Model file for the job. Use its own axes, mm. Face numbers are marked on the shaded views. Round coordinates to 2 decimals unless told otherwise and drop trailing zeros. Order: outer loops, then holes, each group sorted by start corner. A loop starts at its lowest first (then second) coordinate and runs counter-clockwise, first axis right, second up. Notation, with made-up numbers: (46, 83.25) - (92, 83.25) arc R14 ccw to (92, 91.25) - close; hole circle Ø10 at (61, 34). An arc over 180 degrees is marked (long way). Answer as CSV lines item,"result". Start each with the question number.
1. Wall check: line 1 along Y through (x, z) = (1.8, 0) (3 decimals); line 2 along Z through (x, y) = (0.8, 0) (3 decimals); line 3 along Y through (x, z) = (0.3, -1.25). Give the ranges that are in metal, low to high. Write a range as [from, to].
2. Pull direction Z, two halves, no side cores. Call the marked faces 1, 2 and 3: released by +Z, released by -Z, zero draft, split by the parting line, or undercut.
3. Band-saw the part on A-A on x = 1.5. List the corners of the cut face in (y, z) (3 decimals), then the cut area to 3 significant figures.
4. Pin check, flat tips, straight feed: pin 1 Ø1.5 at (x, z) = (1.5, -2) entering from -Y; pin 2 Ø1 at (x, y) = (2, -1.5) entering from -Z. Stop position of each tip, or through.
```python
from build123d import *

# Parameters (mm, degrees)
RESSALTO_EXTRUS_O1_DEPTH = 3
FILETE1_R                = 0.2
ESBO_O12_OUTSIDE_W       = 88.106
ESBO_O12_OUTSIDE_H       = 86.648
ESBO_O12_OUTSIDE_R       = 5
CORTE_EXTRUS_O3_DEPTH    = 13
CORTE_EXTRUS_O3_DRAFT    = -70
ESBO_O17_OUTSIDE_W       = 88.106
ESBO_O17_OUTSIDE_H       = 86.648
ESBO_O17_OUTSIDE_R       = 4.994498725
CORTE_EXTRUS_O4_DEPTH    = 13
CORTE_EXTRUS_O4_DRAFT    = -70


with BuildPart() as part:
    # Esboço1 → Ressalto-extrusão1 (new body)
    with BuildSketch(Plane(origin=(0, 0, 0), x_dir=(0, 0, -1), z_dir=(1, 0, 0))):
        Polygon((2.808721651, 5.044245833), (-2.964084209, 4.954547218), (-5.77280586, -0.089698615), (-2.808721651, -5.044245833), (2.964084209, -4.954547218), (5.77280586, 0.089698615), align=None)
    extrude(amount=RESSALTO_EXTRUS_O1_DEPTH)

    # Esboço11 → Furo roscado de M6x0.752 (revolve, cut)
    with BuildSketch(Plane(origin=(3, 0, 0), x_dir=(0, 0, -1), z_dir=(0, 1, 0))):
        Polygon((0, 0), (0, 3), (2.625, 3), (2.625, 0.4), (3.025, 0), align=None)
    revolve(axis=Axis((9.35, 0, 0), (-1, 0, 0)), mode=Mode.SUBTRACT)

    # Filete1
    filete1_edges = [part.edges().sort_by_distance(p)[0] for p in [
        (0, 0, 2.625),
    ]]
    fillet(filete1_edges, radius=FILETE1_R)


with BuildPart() as corte_extrus_o3_tool:
    # Esboço12 outside → Corte-extrusão3 (with draft: the straight prism first)
    with BuildSketch(Plane(origin=(3, 0, 0), x_dir=(0, 0, -1), z_dir=(1, 0, 0))):
        Rectangle(ESBO_O12_OUTSIDE_W, ESBO_O12_OUTSIDE_H)
        Circle(ESBO_O12_OUTSIDE_R, mode=Mode.SUBTRACT)
    extrude(amount=-CORTE_EXTRUS_O3_DEPTH)
    # Corte-extrusão3: the draft: its side faces are tilted about the plane it starts from
    corte_extrus_o3_sides = [corte_extrus_o3_tool.faces().sort_by_distance(p)[0] for p in [
        (-3.5, -43.324, 0),
        (-3.5, 0, -44.053),
        (-3.5, 43.324, 0),
        (-3.5, 0, 44.053),
        (-3.5, 0, 5),
    ]]
    draft(corte_extrus_o3_sides, Plane(origin=(3, 0, 0), x_dir=(0, 0, -1), z_dir=(1, 0, 0)), CORTE_EXTRUS_O3_DRAFT)


with BuildPart() as part_1:
    add(part.part)

    # Corte-extrusão3: cut by corte_extrus_o3_tool
    add(corte_extrus_o3_tool.part, mode=Mode.SUBTRACT)


with BuildPart() as corte_extrus_o4_tool:
    # Esboço17 outside → Corte-extrusão4 (with draft: the straight prism first)
    with BuildSketch(Plane.ZY):
        Rectangle(ESBO_O17_OUTSIDE_W, ESBO_O17_OUTSIDE_H)
        Circle(ESBO_O17_OUTSIDE_R, mode=Mode.SUBTRACT)
    extrude(amount=-CORTE_EXTRUS_O4_DEPTH)
    # Corte-extrusão4: the draft: its side faces are tilted about the plane it starts from
    corte_extrus_o4_sides = [corte_extrus_o4_tool.faces().sort_by_distance(p)[0] for p in [
        (6.5, -43.324, 0),
        (6.5, 0, 44.053),
        (6.5, 43.324, 0),
        (6.5, 0, -44.053),
        (6.5, 0, -4.994498725),
    ]]
    draft(corte_extrus_o4_sides, Plane.ZY, CORTE_EXTRUS_O4_DRAFT)


with BuildPart() as part_2:
    add(part_1.part)

    # Corte-extrusão4: cut by corte_extrus_o4_tool
    add(corte_extrus_o4_tool.part, mode=Mode.SUBTRACT)


solid = part_2.part
```
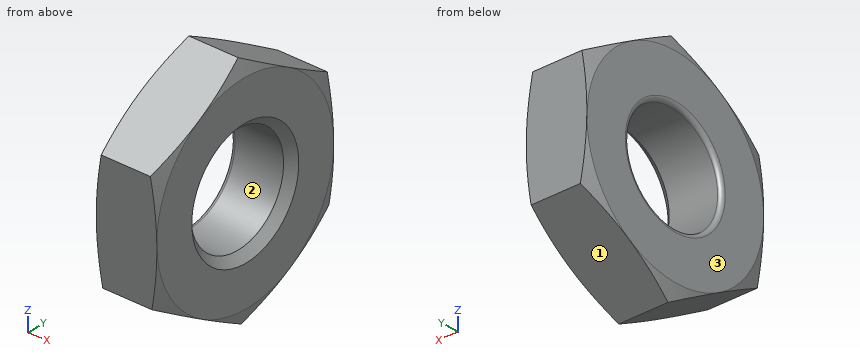
Reply:
1,line 1,"y = [-5.001, -2.625], [2.625, 5.001]"
1,line 2,"z = [-5.723, -2.625], [2.625, 5.723]"
1,line 3,"y = [-4.98, -2.31], [2.31, 5.02]"
2,face 1,"released by -Z"
2,face 2,"undercut"
2,face 3,"zero draft"
3,outline,"(-5.044, 2.809) - (-4.955, -2.964) - (0.09, -5.773) - (5.044, -2.809) - (4.955, 2.964) - (-0.09, 5.773) - close; hole circle Ø5.25 at (0, 0)"
3,area,"65.0 mm2"
4,pin 1,"stops at y = -4.98"
4,pin 2,"stops at z = -5.17"
